Here's how the part is built. I have some questions about the finished solid (model axes, mm). Give positions to 0.01 mm unless a question says otherwise; leave off trailing zeros. Loops run counter-clockwise (first coordinate to the right, second up) from the corner with the lowest first, then second, coordinate; pieces in that order, holes last. Notation, with made-up numbers: M 71,-35 L 127,-35 A24 ccw 127,-25 Z; hole C 28,44 d5. An arc over 180 degrees is marked long. Write item = value, one per line. Start each with the question number.
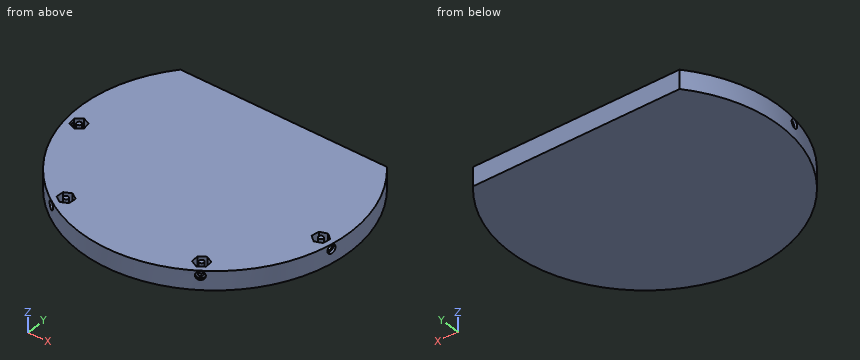
Autodesk Inventor part; units mm, degrees
ref_plane "Work Plane1" through (82.8425, -15.3643, -8) normal (-0.9881, 0.1538, 0) x (0, 0, 1)
ref_plane "Work Plane2" through (44.6398, -71.4579, 0) normal (-0.5541, 0.8324, 0) x (0.8324, 0.5541, 0)
ref_plane "Work Plane3" through (-48.6961, -68.7578, 0) normal (0.5541, 0.8324, 0) x (0.8324, -0.5541, 0)
sketch "Sketch1" plane through (0, 0, 0) normal (0, 0, 1) x (1, 0, 0)
  circle A0 centre (0, 0) radius 85.8
  line L0 (-72.5268, -13.7582) -> (-76.3217, -16.8148)
  line L1 (-76.3217, -16.8148) -> (-80.8663, -15.0566)
  line L2 (-80.8663, -15.0566) -> (-81.616, -10.2418)
  line L3 (-81.616, -10.2418) -> (-77.8211, -7.1852)
  line L4 (-77.8211, -7.1852) -> (-73.2765, -8.9434)
  line L5 (-73.2765, -8.9434) -> (-72.5268, -13.7582)
  line L6 (73.2765, -8.9434) -> (77.8211, -7.1852)
  line L7 (77.8211, -7.1852) -> (81.616, -10.2418)
  line L8 (81.616, -10.2418) -> (80.8663, -15.0566)
  line L9 (80.8663, -15.0566) -> (76.3217, -16.8148)
  line L10 (76.3217, -16.8148) -> (72.5268, -13.7582)
  line L11 (72.5268, -13.7582) -> (73.2765, -8.9434)
  line L12 (-77.0714, -12) -> (0, 0) construction
  line L13 (77.0714, -12) -> (0, 0) construction
  line L14 (0, 0) -> (85.8, 0) construction
  line L15 (47.5879, -67.0929) -> (43.5316, -69.793)
  line L16 (47.2777, -62.2299) -> (47.5879, -67.0929)
  line L17 (42.9111, -60.0671) -> (47.2777, -62.2299)
  line L18 (38.8548, -62.7673) -> (42.9111, -60.0671)
  line L19 (39.165, -67.6302) -> (38.8548, -62.7673)
  line L20 (43.5316, -69.793) -> (39.165, -67.6302)
  line L21 (-47.2777, -62.2299) -> (-42.9111, -60.0671)
  line L22 (-42.9111, -60.0671) -> (-38.8548, -62.7673)
  line L23 (-38.8548, -62.7673) -> (-39.165, -67.6302)
  line L24 (-39.165, -67.6302) -> (-43.5316, -69.793)
  line L25 (-43.5316, -69.793) -> (-47.5879, -67.0929)
  line L26 (-47.5879, -67.0929) -> (-47.2777, -62.2299)
  line L27 (-65.8532, 55) -> (65.8532, 55)
  circle A1 centre (77.0714, -12) radius 1.5
  circle A2 centre (43.2214, -64.9301) radius 1.5
  circle A3 centre (-43.2214, -64.9301) radius 1.5
  circle A4 centre (-77.0714, -12) radius 1.5
  dimension "d0" = 171.6
  dimension "d1" = 78
  dimension "d2" = 78
  dimension "d5" = 12
  dimension "d6" = 4.22
  dimension "d7" = 4.22
  dimension "d10" = 12
  dimension "d13" = 47.5
  dimension "d17" = 47.5
  dimension "d19" = 55
  dimension "d81" = 3
  dimension "d82" = 3
  dimension "d83" = 3
  dimension "d84" = 3
extrude "Extrusion1" add sketch "Sketch1" against normal blind 12 contours A0 L27 | A1 | A2 | A3 | A4 picked at (21.9511, 12.3711)
sketch "Sketch2" plane through (0, 0, -12) normal (0, 0, -1) x (-1, 0, 0)
  arc A0 (-65.8532, 55) -> (65.8532, 55) centre (0, 0) ccw
  line L0 (65.8532, 55) -> (-65.8532, 55)
  line L1 (76.3217, -16.8148) -> (72.5268, -13.7582)
  line L2 (72.5268, -13.7582) -> (73.2765, -8.9434)
  line L3 (73.2765, -8.9434) -> (77.8211, -7.1852)
  line L4 (77.8211, -7.1852) -> (81.616, -10.2418)
  line L5 (81.616, -10.2418) -> (80.8663, -15.0566)
  line L6 (80.8663, -15.0566) -> (76.3217, -16.8148)
  line L7 (-77.8211, -7.1852) -> (-73.2765, -8.9434)
  line L8 (-73.2765, -8.9434) -> (-72.5268, -13.7582)
  line L9 (-72.5268, -13.7582) -> (-76.3217, -16.8148)
  line L10 (-76.3217, -16.8148) -> (-80.8663, -15.0566)
  line L11 (-80.8663, -15.0566) -> (-81.616, -10.2418)
  line L12 (-81.616, -10.2418) -> (-77.8211, -7.1852)
  line L13 (-43.5316, -69.793) -> (-47.5879, -67.0929)
  line L14 (-47.5879, -67.0929) -> (-47.2777, -62.2299)
  line L15 (-47.2777, -62.2299) -> (-42.9111, -60.0671)
  line L16 (-42.9111, -60.0671) -> (-38.8548, -62.7673)
  line L17 (-38.8548, -62.7673) -> (-39.165, -67.6302)
  line L18 (-39.165, -67.6302) -> (-43.5316, -69.793)
  line L19 (42.9111, -60.0671) -> (47.2777, -62.2299)
  line L20 (47.2777, -62.2299) -> (47.5879, -67.0929)
  line L21 (47.5879, -67.0929) -> (43.5316, -69.793)
  line L22 (43.5316, -69.793) -> (39.165, -67.6302)
  line L23 (39.165, -67.6302) -> (38.8548, -62.7673)
  line L24 (38.8548, -62.7673) -> (42.9111, -60.0671)
extrude "Extrusion2" add sketch "Sketch2" against normal blind 4 contours L1 L2 L3 L4 L5 L6 | L7 L8 L9 L10 L11 L12 | L13 L14 L15 L16 L17 L18 | L19 L20 L21 L22 L23 L24
sketch "Sketch3" plane through (80.8663, -15.0566, -8) normal (-0.9881, 0.1538, 0) x (0, 0, 1)
  line L0 (0, 4.8728) -> (0, 0)
  line L1 (8, 0) -> (0, 0)
  line L2 (8, 4.8728) -> (8, 0)
  line L3 (8, 4.8728) -> (0, 4.8728)
  circle A0 centre (5, 2.4364) radius 1.5
  point P0 (8, 2.4364)
  dimension "d24" = 3
  dimension "d26" = 5
  dimension "d27" = 2.4364
extrude "Extrusion3" cut sketch "Sketch3" against normal blind 5 contours A0
sketch "Sketch4" plane through (43.5316, -69.793, 0) normal (-0.5541, 0.8324, 0) x (0.8324, 0.5541, 0)
  line L0 (4.8728, 8) -> (0, 8)
  line L1 (0, 0) -> (0, 8)
  line L2 (4.8728, 0) -> (0, 0)
  line L3 (4.8728, 0) -> (4.8728, 8)
  circle A0 centre (2.4364, 3) radius 1.5
  point P0 (2.4364, 0)
  dimension "d30" = 3
  dimension "d31" = 5
  dimension "d32" = 2.4364
extrude "Extrusion4" cut sketch "Sketch4" against normal blind 5 contours A0
sketch "Sketch5" plane through (-47.5879, -67.0929, 0) normal (0.5541, 0.8324, 0) x (0.8324, -0.5541, 0)
  line L0 (4.8728, 8) -> (0, 8)
  line L1 (0, 0) -> (0, 8)
  line L2 (4.8728, 0) -> (0, 0)
  line L3 (4.8728, 0) -> (4.8728, 8)
  circle A0 centre (2.4364, 3) radius 1.5
  point P0 (2.4364, 0)
  dimension "d35" = 3
  dimension "d36" = 2.4364
  dimension "d37" = 5
extrude "Extrusion5" cut sketch "Sketch5" against normal blind 5 contours A0
sketch "Sketch6" plane through (-81.616, -10.2418, 0) normal (0.9881, 0.1538, 0) x (0, 0, -1)
  line L0 (8, -4.8728) -> (8, 0)
  line L1 (0, 0) -> (8, 0)
  line L2 (0, -4.8728) -> (0, 0)
  line L3 (0, -4.8728) -> (8, -4.8728)
  circle A0 centre (3, -2.4364) radius 1.5
  point P0 (0, -2.4364)
  dimension "d40" = 3
  dimension "d41" = 2.4364
  dimension "d42" = 5
extrude "Extrusion6" cut sketch "Sketch6" against normal blind 5 contours A0
ref_plane "Work Plane1" through (82.8425, -15.3643, -8) normal (-0.9881, 0.1538, 0) x (0, 0, 1)
sketch "Sketch7" plane through (82.8425, -15.3643, -8) normal (-0.9881, 0.1538, 0) x (0, 0, 1)
  circle A0 centre (5, 2.4364) radius 1.5
  circle A1 centre (5, 2.4364) radius 2.75
  point P0 (8, 2.4364)
  dimension "d46" = 5.5
extrude "Extrusion7" cut sketch "Sketch7" against normal up to surface contours A0 | A1
ref_plane "Work Plane2" through (44.6398, -71.4579, 0) normal (-0.5541, 0.8324, 0) x (0.8324, 0.5541, 0)
sketch "Sketch8" plane through (44.6398, -71.4579, 0) normal (-0.5541, 0.8324, 0) x (0.8324, 0.5541, 0)
  circle A0 centre (2.4364, 3) radius 1.5
  circle A1 centre (2.4364, 3) radius 2.75
  point P0 (2.4364, 0)
  dimension "d50" = 5.5
extrude "Extrusion8" cut sketch "Sketch8" against normal up to surface contours A0 | A1
ref_plane "Work Plane3" through (-48.6961, -68.7578, 0) normal (0.5541, 0.8324, 0) x (0.8324, -0.5541, 0)
sketch "Sketch9" plane through (-48.6961, -68.7578, 0) normal (0.5541, 0.8324, 0) x (0.8324, -0.5541, 0)
  circle A0 centre (2.4364, 3) radius 1.5
  circle A1 centre (2.4364, 3) radius 2.75
  point P0 (2.4364, 0)
  dimension "d54" = 5.5
extrude "Extrusion9" cut sketch "Sketch9" against normal up to surface contours A0 | A1
ref_plane "Work Plane4" through (-83.5922, -10.5495, 0) normal (0.9881, 0.1538, 0) x (0, 0, -1)
sketch "Sketch10" plane through (-83.5922, -10.5495, 0) normal (0.9881, 0.1538, 0) x (0, 0, -1)
  circle A0 centre (3, -2.4364) radius 1.5
  circle A1 centre (3, -2.4364) radius 2.75
  point P0 (0, -2.4364)
  dimension "d58" = 5.5
extrude "Extrusion10" cut sketch "Sketch10" against normal up to surface contours A0 | A1
sketch "Sketch11" plane through (0, 0, -12) normal (0, 0, -1) x (-1, 0, 0)
  line L0 (75.3409, 34.7165) -> (17.3409, 34.7165) construction
  line L1 (17.3409, 34.7165) -> (17.3409, -14.2835) construction
  line L2 (17.3409, -14.2835) -> (75.3409, -14.2835) construction
  line L3 (75.3409, -14.2835) -> (75.3409, 34.7165) construction
  circle A0 centre (75.3409, 34.7165) radius 1.5
  circle A1 centre (75.3409, -14.2835) radius 1.5
  circle A2 centre (17.3409, 34.7165) radius 1.5
  circle A3 centre (17.3409, -14.2835) radius 1.5
  line L4 (59.7604, -34.3641) -> (1.7604, -34.3641) construction
  line L5 (1.7604, -34.3641) -> (1.7604, -57.3641) construction
  line L6 (1.7604, -57.3641) -> (59.7604, -57.3641) construction
  line L7 (59.7604, -57.3641) -> (59.7604, -34.3641) construction
  circle A4 centre (59.7604, -34.3641) radius 1.5
  circle A5 centre (59.7604, -57.3641) radius 1.5
  circle A6 centre (1.7604, -57.3641) radius 1.5
  circle A7 centre (1.7604, -34.3641) radius 1.5
  dimension "d69" = 58
  dimension "d70" = 49
  dimension "d71" = 3
  dimension "d72" = 3
  dimension "d73" = 3
  dimension "d74" = 3
  dimension "d75" = 58
  dimension "d76" = 23
  dimension "d77" = 3
  dimension "d78" = 3
  dimension "d79" = 3
  dimension "d80" = 3
properties part number "plate_third_floor"
Q1. If I drill on line 1 along X through (y, z) = (-61.5, -3); line 2 along Y through (x, z) = (-22.5, -0.5); line 3 along Y through (x, z) = (-47, -7.25), over which ranges is the centre line in solid material (lowest first)?
Q2. Will these pins go through, and if not, where does the flat tip stop? pin 1 (2.5 mm diameter, centred on x = -42.5, y = -64.5, fed in from +Z); pin 2 (2 mm diameter, centred on y = -59, z = -4, fed in from +X); pin 3 (6 mm diameter, centred on y = -62, z = -6.5, fed in from -X).
Q3. If we section it at B-B, the plane y = -23: List the corners of the cut face in (x, z) for me.
Q4. If we section it at C-C, the plane z = -10: List the corners of the cut face in (x, y) for me.
Q5. If we section it at A-A, the plane x = 53: List the corners of the cut face in (y, z) for me.
Resolved:
q1.line_1 = -59.83 to -45.8, -40.76 to 40.76, 45.8 to 59.83
q1.line_2 = -82.8 to 55
q1.line_3 = -71.78 to -67.48, -62.09 to 55
q2.pin_1 = 0
q2.pin_2 = 63.23
q2.pin_3 = -62.29
q3.outline = M -82.66,-12 L 82.66,-12 L 82.66,0 L -82.66,0 Z
q4.outline = M -65.85,55 A85.8 ccw long 65.85,55 Z
q5.outline = M -67.47,-12 L 55,-12 L 55,0 L -67.47,0 Z
